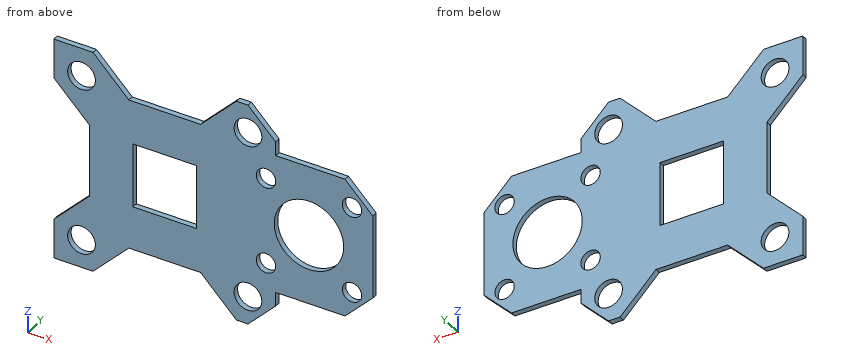
```python
from build123d import *

# Parameters (mm, degrees)
SKETCH1_W           = 80
SKETCH1_H           = 80
BOSS_EXTRUDE1_DEPTH = 2
SKETCH2_R           = 2.5
CUT_EXTRUDE1_DEPTH  = 10
SKETCH4_W           = 80
SKETCH4_H           = 2
BOSS_EXTRUDE2_DEPTH = 35
SKETCH3_R           = 1.5
SKETCH3_R_2         = 12.5
CUT_EXTRUDE2_DEPTH  = 10
SKETCH5_W           = 23
SKETCH5_H           = 23
CUT_EXTRUDE3_DEPTH  = 10
SKETCH6_W           = 35
SKETCH6_H           = 15
CUT_EXTRUDE4_DEPTH  = 10
CHAMFER1_SIZE       = 10
SKETCH7_R           = 5
CUT_EXTRUDE5_DEPTH  = 4
SKETCH8_R           = 3.5
CUT_EXTRUDE6_DEPTH  = 3


with BuildPart() as part:
    # Sketch1 → Boss-Extrude1 (new body)
    with BuildSketch(Plane(origin=(0, 0, 0), x_dir=(1, 0, 0), z_dir=(0, 1, 0))):
        with Locations((40, 40)):
            Rectangle(SKETCH1_W, SKETCH1_H)
    extrude(amount=BOSS_EXTRUDE1_DEPTH)

    # Sketch2 → Cut-Extrude1 (cut)
    with BuildSketch(Plane.XZ):
        with Locations(Location((70, -70, 0), (0, 0, 270))):
            Circle(SKETCH2_R)
        with Locations(Location((70, -10, 0), (0, 0, 270))):
            Circle(SKETCH2_R)
        with Locations(Location((10, -10, 0), (0, 0, 270))):
            Circle(SKETCH2_R)
        with Locations(Location((10, -70, 0), (0, 0, 270))):
            Circle(SKETCH2_R)
    extrude(amount=-CUT_EXTRUDE1_DEPTH, mode=Mode.SUBTRACT)

    # Sketch4 → Boss-Extrude2 (add)
    with BuildSketch(Plane(origin=(80, 0, 0), x_dir=(0, 0, -1), z_dir=(1, 0, 0))):
        with Locations((40, 1)):
            Rectangle(SKETCH4_W, SKETCH4_H)
    extrude(amount=BOSS_EXTRUDE2_DEPTH)

    # Sketch3 → Cut-Extrude2 (cut)
    with BuildSketch(Plane.XZ):
        with Locations(Location((107.5, -24.5, 0), (0, 0, 270))):
            Circle(SKETCH3_R)
        with Locations(Location((107.5, -55.5, 0), (0, 0, 270))):
            Circle(SKETCH3_R)
        with Locations(Location((76.5, -55.5, 0), (0, 0, 270))):
            Circle(SKETCH3_R)
        with Locations(Location((76.5, -24.5, 0), (0, 0, 270))):
            Circle(SKETCH3_R)
        with Locations(Location((92, -40, 0), (0, 0, 270))):
            Circle(SKETCH3_R_2)
    extrude(amount=-CUT_EXTRUDE2_DEPTH, mode=Mode.SUBTRACT)

    # Sketch5 → Cut-Extrude3 (cut)
    with BuildSketch(Plane(origin=(0, 2, 0), x_dir=(1, 0, 0), z_dir=(0, 1, 0))):
        Polygon((65.857864376, 80), (14.142135624, 80), (27.071067812, 67.071067812), (52.928932188, 67.071067812), align=None)
        with Locations((40, 40)):
            Rectangle(SKETCH5_W, SKETCH5_H)
        Polygon((27.071067812, 12.928932188), (14.142135624, 0), (65.857864376, 0), (52.928932188, 12.928932188), align=None)
        Polygon((12.928932188, 52.928932188), (0, 65.857864376), (0, 14.142135624), (12.928932188, 27.071067812), align=None)
    extrude(amount=-CUT_EXTRUDE3_DEPTH, mode=Mode.SUBTRACT)

    # Sketch6 → Cut-Extrude4 (cut)
    with BuildSketch(Plane(origin=(0, 2, 0), x_dir=(1, 0, 0), z_dir=(0, 1, 0))):
        with Locations((97.5, 72.5)):
            Rectangle(SKETCH6_W, SKETCH6_H)
        with Locations((97.5, 7.5)):
            Rectangle(SKETCH6_W, SKETCH6_H)
    extrude(amount=-CUT_EXTRUDE4_DEPTH, mode=Mode.SUBTRACT)

    # Chamfer1
    chamfer1_edges = [part.edges().sort_by_distance(p)[0] for p in [
        (115, 1, -15),
        (115, 1, -65),
        (80, 1, -80),
        (80, 1, 0),
    ]]
    chamfer(chamfer1_edges, length=CHAMFER1_SIZE)

    # Sketch7 → Cut-Extrude5 (cut)
    with BuildSketch(Plane(origin=(0, 2, 0), x_dir=(1, 0, 0), z_dir=(0, 1, 0))):
        with Locations(Location((70, 70, 0), (0, 0, 270))):
            Circle(SKETCH7_R)
        with Locations(Location((70, 10, 0), (0, 0, 270))):
            Circle(SKETCH7_R)
        with Locations(Location((10, 10, 0), (0, 0, 270))):
            Circle(SKETCH7_R)
        with Locations(Location((10, 70, 0), (0, 0, 270))):
            Circle(SKETCH7_R)
    extrude(amount=-CUT_EXTRUDE5_DEPTH, mode=Mode.SUBTRACT)

    # Sketch8 → Cut-Extrude6 (cut)
    with BuildSketch(Plane.XZ):
        with Locations(Location((107.5, -24.5, 0), (0, 0, 270))):
            Circle(SKETCH8_R)
        with Locations(Location((107.5, -55.5, 0), (0, 0, 270))):
            Circle(SKETCH8_R)
        with Locations(Location((76.5, -55.5, 0), (0, 0, 270))):
            Circle(SKETCH8_R)
        with Locations(Location((76.5, -24.5, 0), (0, 0, 270))):
            Circle(SKETCH8_R)
    extrude(amount=-CUT_EXTRUDE6_DEPTH, mode=Mode.SUBTRACT)


solid = part.part
```
Here's how the part is built. I have some questions about the finished solid (model axes, mm). Round coordinates to 2 decimals unless told otherwise and drop trailing zeros. Loops run counter-clockwise (first coordinate to the right, second up) from the corner with the lowest first, then second, coordinate; pieces in that order, holes last.
1. Will these pins go through, and if not, where does the flat tip stop? pin 1 (0.6 mm diameter, centred on x = 37.5, y = 1.5, fed in from +Z); pin 2 (1 mm diameter, centred on y = 0.5, z = -41, fed in from -X); pin 3 (1 mm diameter, centred on y = 1.5, z = -68.5, fed in from +X).
Answers:
pin 1: stops at z = -12.93
pin 2: stops at x = 12.93
pin 3: stops at x = 80
2. If I drill on probe 1 along X at (y, z) = (0.95, -14); probe 2 along X at (y, z) = (1.1, -40); probe 3 along X at (y, z) = (1.15, -6), over which ranges is the centre line in solid material (lowest first)?
Answers:
probe 1: x = 0 to 7, 13 to 67, 73 to 80
probe 2: x = 12.93 to 28.5, 51.5 to 79.5, 104.5 to 115
probe 3: x = 0 to 7, 13 to 20.14, 59.86 to 67, 73 to 76
3. Suppose I cut it at B-B, the plane x = 43. Please give me the cut outline in (y, z), and give its area (3 significant figures).
Answers:
outline: (0, -67.07) - (2, -67.07) - (2, -51.5) - (0, -51.5) - close; (0, -28.5) - (2, -28.5) - (2, -12.93) - (0, -12.93) - close
area: 62.3 mm2
4. Suppose I cut it at D-D, the plane y = 1.4. Give the number of separate pieces and of enclosed holes in the cut face, and give its area (3 significant figures).
Answers:
separate pieces: 1
enclosed holes: 10
area: 4,960 mm2
5. Suppose I cut it at C-C, the plane z = -71.5. Please give me the cut outline in (x, y), and give its area (3 significant figures).
Answers:
outline: (0, 0) - (5.23, 0) - (5.23, 2) - (0, 2) - close; (14.77, 0) - (22.64, 0) - (22.64, 2) - (14.77, 2) - close; (57.36, 0) - (65.23, 0) - (65.23, 2) - (57.36, 2) - close; (74.77, 0) - (78.5, 0) - (78.5, 2) - (74.77, 2) - close
area: 49.4 mm2
6. Suppose I cut it at A-A, the plane x = 107.5. Please give me the cut outline in (y, z), and give its area (3 significant figures).
Answers:
outline: (0, -62.5) - (2, -62.5) - (2, -59) - (0, -59) - close; (0, -52) - (2, -52) - (2, -28) - (0, -28) - close; (0, -21) - (2, -21) - (2, -17.5) - (0, -17.5) - close
area: 62.0 mm2
